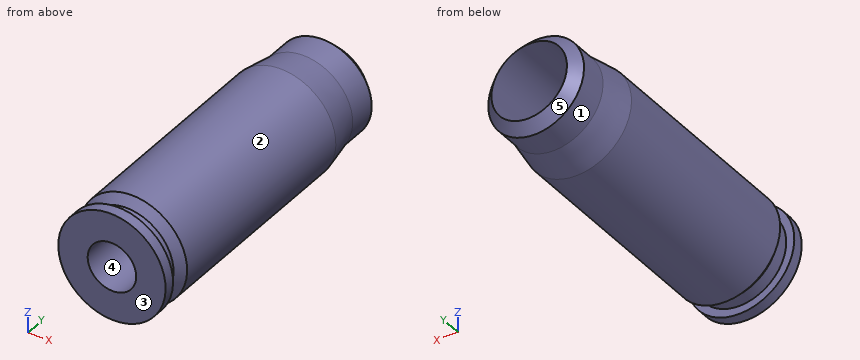
```python
from build123d import *

# Parameters (mm, degrees)
CHAMFER_1_SIZE = 3


with BuildPart() as part:
    # 스케치3 → 회전1 (revolve)
    with BuildSketch(Plane(origin=(0, 0, 0), x_dir=(0, 0, -1), z_dir=(1, 0, 0))):
        Polygon((4.5, 0), (9.95, 0), (9.95, 2), (8.458613311, 2), (8.458613311, 4.3), (9.95, 5.791386689), (9.95, 45.791386689), (8.875, 51.888014645), (8.875, 60), (7, 60), (7, 12), (4.5, 12), align=None)
    revolve(axis=Axis((0, 0, 0), (0, 1, 0)))

    # 모따기1
    # the kernel refuses this chamfer: 3 mm, written as the material it takes off along each edge
    with BuildSketch(Plane(origin=(0, 60, 0), x_dir=(0, 0, -1), z_dir=(1, 0, 0))) as chamfer_1_piece_1:
        Polygon((8.875, -CHAMFER_1_SIZE), (8.875 - CHAMFER_1_SIZE, 0), (8.875, 0), align=None)
    revolve(axis=Axis((0, 60, 0), (0, 1, 0)), mode=Mode.SUBTRACT)


solid = part.part
```
Geometry: final body of the model. Coordinates: model frame, mm. Face numbers are marked on the shaded views. A direction names the side the tool comes from. Give positions to 0.01 mm unless a question says otherwise; leave off trailing zeros. Order: outer loops, then holes, each group sorted by start corner. A loop starts at its lowest first (then second) coordinate and runs counter-clockwise, first axis right, second up. Notation, with made-up numbers: M 62,40.25 L 84,40.25 A29 ccw 84,75.25 Z; hole C 86,39.25 d7. An arc over 180 degrees is marked long. Answer as CSV lines item,"result". Start each with the question number.
1) Set-up query: the marked faces 1 and 2. Return all of +Z, -Z, +X, -X, +Y, -Y with unobstructed straight access to the full face (end or side cutting, diameter ignored); none if empty.
2) First-contact query: P1, Ø1.5, axis at x = 5, y = 41, coming from the +Z side; P2, Ø4, axis at y = 52.5, z = 0, coming from the +X side; P3, Ø1.5, axis at x = -2.5, y = 31, coming from the +Z side. Flat tips, straight axial feed; report the tip coordinate or a pass-through.
3) Line query: line 1 (X direction, y = 40, z = 0); line 2 (Z direction, x = 0, y = 8); line 3 (Z direction, x = 0, y = 3.25). Output: solid intervals per line, ascending. Write a range as from..to.
4) Cut plane A-A (z = 0). Output: boundary loops of the cut face in (x, y) (3 decimals), then the cut area to 3 significant figures.
5) Mould query, pull axis X, two halves, no side actions, for the marked faces 3, 4 and 5. Classes: +X half, -X half, draft (parallel to the pull), parting line (faces both ways), or undercut.
6) Cut plane C-C (y = 7.5). Output: boundary loops of the cut face in (x, z), then the cut area to 3 significant figures.
7) Cut plane D-D (y = 32.5). Output: boundary loops of the cut face in (x, z), then the cut area to 3 significant figures.
8) Cut plane B-B (x = 0). Output: boundary loops of the cut face in (y, z) (3 decimals).
Findings below:
1,face 1,"+Y"
1,face 2,"+Y, -Y"
2,P1,"stops at z = 9"
2,P2,"stops at x = 9.12"
2,P3,"stops at z = 9.79"
3,line 1,"x = -9.95..-7, 7..9.95"
3,line 2,"z = -9.95..-4.5, 4.5..9.95"
3,line 3,"z = -8.46..-4.5, 4.5..8.46"
4,outline,"M -9.95,0 L -4.5,0 L -4.5,12 L -7,12 L -7,58.875 L -8.875,57 L -8.875,51.888 L -9.95,45.791 L -9.95,5.791 L -8.459,4.3 L -8.459,2 L -9.95,2 Z; M 4.5,0 L 9.95,0 L 9.95,2 L 8.459,2 L 8.459,4.3 L 9.95,5.791 L 9.95,45.791 L 8.875,51.888 L 8.875,57 L 7,58.875 L 7,12 L 4.5,12 Z"
4,area,"373 mm²"
5,face 3,"draft"
5,face 4,"undercut"
5,face 5,"parting line"
6,outline,"C 0,0 d19.9; hole C 0,0 d9"
6,area,"247 mm²"
7,outline,"C 0,0 d19.9; hole C 0,0 d14"
7,area,"157 mm²"
8,outline,"M 0,-9.95 L 2,-9.95 L 2,-8.459 L 4.3,-8.459 L 5.791,-9.95 L 45.791,-9.95 L 51.888,-8.875 L 57,-8.875 L 58.875,-7 L 12,-7 L 12,-4.5 L 0,-4.5 Z; M 0,4.5 L 12,4.5 L 12,7 L 58.875,7 L 57,8.875 L 51.888,8.875 L 45.791,9.95 L 5.791,9.95 L 4.3,8.459 L 2,8.459 L 2,9.95 L 0,9.95 Z"
